Build history of the part. All positions in model axes, mm. A direction names the side the tool comes from. Round coordinates to 2 decimals unless told otherwise and drop trailing zeros. Write each loop counter-clockwise with the first axis right and the second up, starting at its lowest first coordinate (ties: lowest second). Pieces come first, ordered by that corner, then holes. Notation, with made-up numbers: (-8.5, 51.5) -> (48.5, 51.5) arc R17 ccw to (48.5, 55.5) -> close; hole circle Ø11 at (76, 42.5). An arc over 180 degrees is marked (long way). Answer as CSV lines item,"result".
from build123d import *

# Parameters (mm, degrees)
F0_R     = 22.5
F1_DEPTH = 3
F0_R_2   = 25
F2_DEPTH = 8
F3_R     = 5
F4_SIZE2 = 2.3
F4_SIZE  = 1
F5_D     = 5


with BuildPart() as f1:
    # F0 (on Top) → F1 (new body)
    with BuildSketch(Plane.XY):
        Circle(F0_R)
    extrude(amount=F1_DEPTH)

    # F0 (on Top) → F2 (join)
    with BuildSketch(Plane.XY):
        Circle(F0_R_2)
        Circle(F0_R, mode=Mode.SUBTRACT)
    extrude(amount=F2_DEPTH)

    # F3
    f3_edges = [f1.edges().sort_by_distance(p)[0] for p in [
        (-25, 0, 0),
    ]]
    fillet(f3_edges, radius=F3_R)

    # F4
    f4_edges = [f1.edges().sort_by_distance(p)[0] for p in [
        (-22.5, 0, 8),
    ]]
    f4_side = f1.faces().sort_by_distance((-22.5, 0, 5.5))[0]
    chamfer(f4_edges, length=F4_SIZE, length2=F4_SIZE2, reference=f4_side)

    # F5 (through all)
    with Locations(Plane(origin=(0, 0, 0), x_dir=(1, 0, 0), z_dir=(0, 0, -1))):
        with Locations((0, 0)):
            Hole(F5_D / 2)


solid = f1.part
1. Cut at A-A, the plane y = 0. Write the cut outline in (x, z), then the cut area to 3 significant figures.
Results found:
outline,"(-25, 5) arc R5 ccw to (-20, 0) -> (-2.5, 0) -> (-2.5, 3) -> (-22.5, 3) -> (-22.5, 7) -> (-24.8, 8) -> (-25, 8) -> close; (2.5, 0) -> (20, 0) arc R5 ccw to (25, 5) -> (25, 8) -> (24.8, 8) -> (22.5, 7) -> (22.5, 3) -> (2.5, 3) -> close"
area,"147 mm2"
2. Drop flat-ended pins along their axis: pin 1 Ø4 at (x, z) = (-5, 3.5) entering from -Y; pin 2 Ø1.5 at (x, z) = (18, 3) entering from +Y; pin 3 Ø1.5 at (y, z) = (6.5, 6) entering from -X. Give the stop position or say it passes through.
Results found:
pin 1,"stops at y = -24.76"
pin 2,"stops at y = 17.62"
pin 3,"stops at x = -24.33"
3. Cut at D-D, the plane z = 1. Write the cut outline in (x, y), then the cut area to 3 significant figures.
Results found:
outline,"circle Ø46 at (0, 0); hole circle Ø5 at (0, 0)"
area,"1,640 mm2"
4. Which spindle directions (+Z, -Z, +X, -X, +Y, -Y) get a long thin tool onto all of the face, cutting with end or side? Do faces 1 (the cylindrical face through (0.54, 2.44, 1.52)), 2 (the cylindrical face through (10.382, -19.961, 4.972)). Say none if no direction does.
Results found:
face 1,"+Z, -Z"
face 2,"+Z"
5. Cut at C-C, the plane z = 6. Write the cut outline in (x, y).
Results found:
outline,"circle Ø50 at (0, 0); hole circle Ø45 at (0, 0)"
6. Probe line 1 along X through (y, z) = (0.5, 5.75) (3 decimals); line 2 along Y through (x, z) = (0, 4.8); line 3 along Z through (x, y) = (2, 7.5). List the from-to ranges inside material, lowest first.
Results found:
line 1,"x = -24.995 to -22.494, 22.494 to 24.995"
line 2,"y = -25 to -22.5, 22.5 to 25"
line 3,"z = 0 to 3"
7. Mould opens along X. For faces 3 (the flat face through (0, -5, 3)), 4 (the flat face through (4, 0, 0)), 5 (the cylindrical face through (23.846, 7.509, 6.479)) say: +X half, -X half, draft (parallel to the pull), parting line (faces both ways), or undercut.
Results found:
face 3,"undercut"
face 4,"draft"
face 5,"parting line"
